from build123d import *

# Parameters (mm, degrees)
SKETCH_1_W      = 71
SKETCH_1_H      = 41
EXTRUDE_1_DEPTH = 1.5
SKETCH_2_W      = 71
SKETCH_2_H      = 41
SKETCH_2_W_2    = 68
SKETCH_2_H_2    = 38
EXTRUDE_2_DEPTH = 10
SKETCH_3_W      = 100
SKETCH_3_H      = 20
EXTRUDE_3_DEPTH = 1.5


with BuildPart() as part:
    # 草图1 → 凸台-拉伸1 (new body)
    with BuildSketch(Plane(origin=(0, 0, 0), x_dir=(1, 0, 0), z_dir=(0, 1, 0))):
        with Locations((35.5, -20.5)):
            Rectangle(SKETCH_1_W, SKETCH_1_H)
    extrude(amount=EXTRUDE_1_DEPTH)

    # 草图2 → 凸台-拉伸2 (add)
    with BuildSketch(Plane(origin=(0, 1.5, 0), x_dir=(1, 0, 0), z_dir=(0, 1, 0))):
        with Locations((35.5, -20.5)):
            Rectangle(SKETCH_2_W, SKETCH_2_H)
        with Locations((35.5, -20.5)):
            Rectangle(SKETCH_2_W_2, SKETCH_2_H_2, mode=Mode.SUBTRACT)
    extrude(amount=EXTRUDE_2_DEPTH)

    # 草图3 → 凸台-拉伸3 (add)
    with BuildSketch(Plane(origin=(0, 0, 0), x_dir=(-1, 0, 0), z_dir=(0, -1, 0))):
        with Locations((-34.5, -46.5)):
            Rectangle(SKETCH_3_W, SKETCH_3_H)
    extrude(amount=-EXTRUDE_3_DEPTH)


solid = part.part
Could you check a few things on this model? Use its own coordinates, in mm. A direction names the side the tool comes from. Coordinates: 2 decimals unless noted, no trailing zeros. Order: outer loops, then holes, each group sorted by start corner. A loop starts at its lowest first (then second) coordinate and runs counter-clockwise, first axis right, second up.
Q1. Which directions (+Z, -Z, +X, -X, +Y, -Y) give clear straight access to the entire face, cutting with the end or side of a thin tool? Please do faces 5 (the flat face through (1.5, 6, 21)), 6 (the flat face through (33, 11.5, 40)).
Q2. Please list where these lines run through material, in increasing order: L1, parallel to Z at x = 38.5, y = 10.5; L2, parallel to X at y = 8.5, z = 14.5; L3, parallel to Y at x = 6.5, z = 29.5.
Q3. Suppose I cut it at D-D on z = 37.5. Please give me the cut outline in (x, y), and give its area (3 significant figures).
Q4. Will these pins go through, and if not, where does the flat tip stop? pin 1 (10 mm diameter, centred on x = 50, z = 15, fed in from +Y); pin 2 (1.5 mm diameter, centred on y = 7.5, z = 32.5, fed in from -X); pin 3 (3 mm diameter, centred on x = 41, y = 7, fed in from +Z).
Q5. Thinking about a two-plate mould opening in Z: for faces 1 (the flat face through (35, 6, 0)), 2 (the flat face through (35, 6, 41)), 3 (the flat face through (35, 6, 1.5)), 4 (the flat face through (71, 6, 21)), which applies, released by +Z, released by -Z, zero draft, split by the parting line, or undercut?
Q6. Suppose I cut it at B-B on z = 19.5. Please give me the cut outline in (x, y), and give its area (4 significant figures).
Q7. Suppose I cut it at A-A on y = 5.25. Please give me the cut outline in (x, z), and give its area (3 significant figures).
Q8. Suppose I cut it at C-C on x = 29.5. Please give me the cut outline in (y, z), and give its area (3 significant figures).
Answer:
1. face 5: +Y
1. face 6: +Z, -Z, +X, -X, +Y
2. L1: z = 0 to 1.5, 39.5 to 41
2. L2: x = 0 to 1.5, 69.5 to 71
2. L3: y = 0 to 1.5
3. outline: (-15.5, 0) - (84.5, 0) - (84.5, 1.5) - (71, 1.5) - (71, 11.5) - (69.5, 11.5) - (69.5, 1.5) - (1.5, 1.5) - (1.5, 11.5) - (0, 11.5) - (0, 1.5) - (-15.5, 1.5) - close
3. area: 180 mm2
4. pin 1: stops at y = 1.5
4. pin 2: stops at x = 0
4. pin 3: stops at z = 41
5. face 1: released by -Z
5. face 2: released by +Z
5. face 3: undercut
5. face 4: zero draft
6. outline: (0, 0) - (71, 0) - (71, 11.5) - (69.5, 11.5) - (69.5, 1.5) - (1.5, 1.5) - (1.5, 11.5) - (0, 11.5) - close
6. area: 136.5 mm2
7. outline: (0, 0) - (71, 0) - (71, 41) - (0, 41) - close; hole (1.5, 1.5) - (69.5, 1.5) - (69.5, 39.5) - (1.5, 39.5) - close
7. area: 327 mm2
8. outline: (0, 0) - (11.5, 0) - (11.5, 1.5) - (1.5, 1.5) - (1.5, 39.5) - (11.5, 39.5) - (11.5, 41) - (1.5, 41) - (1.5, 56.5) - (0, 56.5) - close
8. area: 115 mm2
